Geometry: final body of the model. Coordinates: model frame, mm. Round coordinates to 2 decimals unless told otherwise and drop trailing zeros. Loops run counter-clockwise (first coordinate to the right, second up) from the corner with the lowest first, then second, coordinate; pieces in that order, holes last. Notation, with made-up numbers: M -29.75,38.5 L -8.75,38.5 A9 ccw -8.75,43.5 Z; hole C 69.25,74.25 d3. An arc over 180 degrees is marked long. Write each question's results on one line, items separated by ' | '.
```python
from build123d import *


with BuildPart() as part:
    # Sketch1 → Revolve1 (revolve)
    with BuildSketch(Plane.XY, mode=Mode.PRIVATE) as revolve1_sk:
        with BuildLine():
            Line((2.15, 0.4), (3, 0.709374699))
            Line((3, 0.709374699), (3, 0.28370359))
            Line((3, 0.28370359), (2.286808057, 0.024122952))
            ThreePointArc((2.286808057, 0.024122952), (2.219459271, 0.006076899), (2.15, 0))
            Line((2.15, 0), (1.4, 0))
            Line((1.4, 0), (1.4, 0.4))
            Line((1.4, 0.4), (2.15, 0.4))
        make_face()
    revolve(revolve1_sk.sketch.rotate(Axis((0, 0, 0), (0, 1, 0)), 90), axis=Axis((0, 0, 0), (0, 1, 0)))  # turned: the seam where the file's is


solid = part.part
```
1. Ray query, probe 1 along X at (y, z) = (0.35, 0); probe 2 along Y at (x, z) = (0.55, 1.6); probe 3 along Y at (x, z) = (-2.2, 1.4). Return the intervals inside material, ascending.
Answer key:
probe 1: x = -3 to -1.4, 1.4 to 3 | probe 2: y = 0 to 0.4 | probe 3: y = 0.14 to 0.57
2. Section A-A (z = 0). Output: boundary loops of the cut face in (x, y), then the cut area to 3 significant figures.
Answer key:
outline: M -3,0.28 L -2.29,0.02 A0.4 ccw -2.15,0 L -1.4,0 L -1.4,0.4 L -2.15,0.4 L -3,0.71 Z; M 1.4,0 L 2.15,0 A0.4 ccw 2.29,0.02 L 3,0.28 L 3,0.71 L 2.15,0.4 L 1.4,0.4 Z | area: 1.32 mm²
3. Draft query along X for faces 1 (the face through (-0.06, 0.2, 1.4)), 2 (the face through (-0.9, 0.49, -2.86)). Return one class per face: pulls with the +X half, pulls with the -X half, needs draft (parallel to the pull), parting line crosses it, or undercut.
Answer key:
face 1: undercut | face 2: parting line crosses it
4. Section B-B (y = 0.6). Output: boundary loops of the cut face in (x, z), then the cut area to 3 significant figures.
Answer key:
outline: C 0,0 d6; hole C 0,0 d5.4 | area: 5.38 mm²
5. Pin query (flat end, axial travel): P1, Ø1.3, axis at x = -0.5, z = -1, coming from the +Y side; P2, Ø2.5, axis at x = 0, z = 0, coming from the +Y side. Return the tip coordinate at first contact, or that it passes through.
Answer key:
P1: stops at y = 0.4 | P2: passes through
6. Section C-C (y = 0.2). Output: boundary loops of the cut face in (x, z).
Answer key:
outline: C 0,0 d5.54; hole C 0,0 d2.8
